Study the drawing (mm; zero at the part's minimum x, y, z) and answer. Coordinates: 2 decimals unless noted, no trailing zeros. Loops run counter-clockwise (first coordinate to the right, second up) from the corner with the lowest first, then second, coordinate; pieces in that order, holes last. Notation, with made-up numbers: (-15.75, 9.5) -> (7.25, 9.5) arc R30 cw to (7.25, 46.5) -> close; hole circle Ø10 at (88.25, 16). An arc over 180 degrees is marked (long way). Answer in a Markdown table with one row per item.
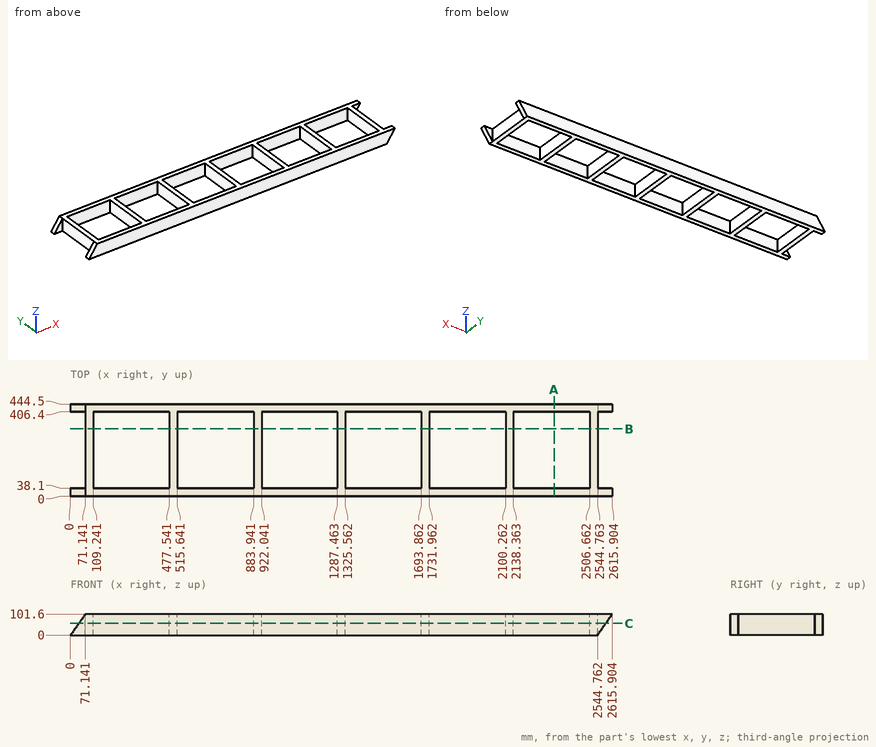
1. A cutting plane is placed at A-A on x = 2334. Give the vertices of the cut face in (y, z).
A:
| item | result |
|---|---|
| outline | (0, 0) -> (38.1, 0) -> (38.1, 101.6) -> (0, 101.6) -> close; (406.4, 0) -> (444.5, 0) -> (444.5, 101.6) -> (406.4, 101.6) -> close |
2. Find the intervals of material crossed by probe 1 along Y at (x, z) = (1956.5, 15.5), in increasing order.
A:
| item | result |
|---|---|
| probe 1 | y = 0 to 38.1, 406.4 to 444.5 |
3. Given pin 1 Ø8 at (y, z) = (229, 12) entering from +X; pin 2 Ø4 at (y, z) = (324, 48.5) entering from -X, each flat-ended and moving along its own axis, determine where each tip first touches the part or whether it passes through.
A:
| item | result |
|---|---|
| pin 1 | stops at x = 2544.76 |
| pin 2 | stops at x = 71.14 |
4. A cutting plane is placed at B-B on y = 324.5. Give the vertices of the cut face in (x, z).
A:
| item | result |
|---|---|
| outline | (71.14, 0) -> (109.24, 0) -> (109.24, 101.6) -> (71.14, 101.6) -> close; (477.54, 0) -> (515.64, 0) -> (515.64, 101.6) -> (477.54, 101.6) -> close; (883.94, 0) -> (922.04, 0) -> (922.04, 101.6) -> (883.94, 101.6) -> close; (1287.46, 0) -> (1325.56, 0) -> (1325.56, 101.6) -> (1287.46, 101.6) -> close; (1693.86, 0) -> (1731.96, 0) -> (1731.96, 101.6) -> (1693.86, 101.6) -> close; (2100.26, 0) -> (2138.36, 0) -> (2138.36, 101.6) -> (2100.26, 101.6) -> close; (2506.66, 0) -> (2544.76, 0) -> (2544.76, 101.6) -> (2506.66, 101.6) -> close |
5. A cutting plane is placed at C-C on z = 56.5. Count the separate pieces of the cut face and the enclosed holes in it, and give its area (3 significant figures).
A:
| item | result |
|---|---|
| separate pieces | 1 |
| enclosed holes | 6 |
| area | 292,000 mm2 |
